```python
from build123d import *

# Parameters (mm, degrees)
SKETCH1_W           = 10
SKETCH1_H           = 10
BOSS_EXTRUDE1_DEPTH = 10
SKETCH2_R           = 1
CUT_EXTRUDE1_DEPTH  = 11
SKETCH3_R           = 1
CUT_EXTRUDE2_DEPTH  = 11
SKETCH5_R           = 1
CUT_EXTRUDE4_DEPTH  = 11
CHAMFER1_SIZE       = 0.2
CHAMFER2_SIZE       = 0.2


with BuildPart() as part:
    # Sketch1 → Boss-Extrude1 (new body)
    with BuildSketch(Plane.XY):
        Rectangle(SKETCH1_W, SKETCH1_H)
    extrude(amount=BOSS_EXTRUDE1_DEPTH)

    # Sketch2 → Cut-Extrude1 (cut, through all)
    with BuildSketch(Plane.XY.offset(10)):
        with Locations((-2.5, 0)):
            Circle(SKETCH2_R)
        with Locations(Location((2.5, 0, 0), (0, 0, 180))):  # turned: the seam where the file's is
            Circle(SKETCH2_R)
    extrude(amount=-CUT_EXTRUDE1_DEPTH, mode=Mode.SUBTRACT)

    # Sketch3 → Cut-Extrude2 (cut, through all)
    with BuildSketch(Plane(origin=(0, 5, 0), x_dir=(1, 0, 0), z_dir=(0, 1, 0))):
        with Locations(Location((0, -7.5, 0), (0, 0, 90))):  # turned: the seam where the file's is
            Circle(SKETCH3_R)
        with Locations(Location((0, -2.5, 0), (0, 0, 270))):  # turned: the seam where the file's is
            Circle(SKETCH3_R)
    extrude(amount=-CUT_EXTRUDE2_DEPTH, mode=Mode.SUBTRACT)

    # Sketch5 → Cut-Extrude4 (cut, through all)
    with BuildSketch(Plane(origin=(5, 0, 0), x_dir=(0, 0, -1), z_dir=(1, 0, 0))):
        with Locations(Location((-5, 2.5, 0), (0, 0, 90))):  # turned: the seam where the file's is
            Circle(SKETCH5_R)
        with Locations(Location((-5, -2.5, 0), (0, 0, 270))):  # turned: the seam where the file's is
            Circle(SKETCH5_R)
    extrude(amount=-CUT_EXTRUDE4_DEPTH, mode=Mode.SUBTRACT)

    # Chamfer1
    chamfer1_edges = [part.edges().sort_by_distance(p)[0] for p in [
        (5, 0, 10),
        (0, 5, 10),
        (-5, 0, 10),
        (0, 5, 0),
        (5, 0, 0),
        (0, -5, 0),
        (-5, 0, 0),
        (0, -5, 10),
        (-5, 5, 5),
        (5, 5, 5),
        (5, -5, 5),
        (-5, -5, 5),
    ]]
    chamfer(chamfer1_edges, length=CHAMFER1_SIZE)

    # Chamfer2
    chamfer2_edges = [part.edges().sort_by_distance(p)[0] for p in [
        (-3.5, 0, 0),
        (-3.5, 0, 10),
        (3.5, 0, 0),
        (3.5, 0, 10),
        (0, -5, 8.5),
        (0, 5, 8.5),
        (0, -5, 1.5),
        (0, 5, 1.5),
        (-5, 1.5, 5),
        (5, 1.5, 5),
        (-5, -1.5, 5),
        (5, -1.5, 5),
    ]]
    chamfer(chamfer2_edges, length=CHAMFER2_SIZE)


solid = part.part
```
Source: CAD feature listing. Evaluate the final solid. Frame: model axes, mm. Round coordinates to 2 decimals unless told otherwise and drop trailing zeros. Loops run counter-clockwise (first coordinate to the right, second up) from the corner with the lowest first, then second, coordinate; pieces in that order, holes last. Notation, with made-up numbers: M 62.25,56.25 L 82.25,56.25 A25 ccw 82.25,75.25 Z; hole C -18,67 d10. An arc over 180 degrees is marked long. Use a Markdown table: item, result. Add a question column.
1. Section query B-B on z = 7.5. Return the cut outline in (x, y), then the cut area to 3 significant figures.
2. Section query A-A on x = 2.5. Return the cut outline in (y, z).
3. Line query: line 1 (Z direction, x = -2, y = -2.5); line 2 (X direction, y = 2.5, z = 7.5); line 3 (X direction, y = 0.5, z = 5.5). Output: solid intervals per line, ascending.
4. Mould query, pull axis Y, two halves, no side actions, for faces 1 (the flat face through (0, 5, 5)), 2 (the cylindrical face through (0.067, -1.763, 4.324)), 3 (the cylindrical face through (-3.3, -0.6, 5.1)), 4 (the flat face through (5, 0, 5)). Classes: pulls with the +Y half, pulls with the -Y half, needs draft (parallel to the pull), parting line crosses it, or undercut.
5. Section query C-C on z = 5.25. Give the number of separate pieces and of enclosed holes in the cut face, then the cut area to 3 significant figures.
Reported:
| question | item | result |
|---|---|---|
| 1 | outline | M -5,-4.8 L -4.8,-5 L -1.2,-5 L -1,-4.8 L -1,4.8 L -1.2,5 L -4.8,5 L -5,4.8 Z; M 1,-4.8 L 1.2,-5 L 4.8,-5 L 5,-4.8 L 5,4.8 L 4.8,5 L 1.2,5 L 1,4.8 Z; hole C -2.5,0 d2; hole C 2.5,0 d2 |
| 1 | area | 73.6 mm² |
| 2 | outline | M -5,0.2 L -4.8,0 L -1.2,0 L -1,0.2 L -1,9.8 L -1.2,10 L -4.8,10 L -5,9.8 Z; M 1,0.2 L 1.2,0 L 4.8,0 L 5,0.2 L 5,9.8 L 4.8,10 L 1.2,10 L 1,9.8 Z; hole C -2.5,5 d2; hole C 2.5,5 d2 |
| 3 | line 1 | z = 0 to 4, 6 to 10 |
| 3 | line 2 | x = -5 to -1, 1 to 5 |
| 3 | line 3 | x = -5 to -3.37, -1.63 to 1.63, 3.37 to 5 |
| 4 | face 1 | pulls with the +Y half |
| 4 | face 2 | undercut |
| 4 | face 3 | undercut |
| 4 | face 4 | needs draft |
| 5 | separate pieces | 3 |
| 5 | enclosed holes | 2 |
| 5 | area | 54.7 mm² |
